Here's how the part is built. I have some questions about the finished solid (model axes, mm). A direction names the side the tool comes from. Give positions to 0.01 mm unless a question says otherwise; leave off trailing zeros. Loops run counter-clockwise (first coordinate to the right, second up) from the corner with the lowest first, then second, coordinate; pieces in that order, holes last.
Q1. Suppose I cut it at C-C (x = -15.5). List the corners of the cut face in (y, z) for me, and give its area (3 significant figures).
Q2. I need wall thicknesses on probe 1 along Y at (x, z) = (-25, 2.2); probe 2 along Y at (x, z) = (-15.5, 0.3); probe 3 along X at (y, z) = (34, 2.4) (3 decimals). Which ranges of each line are inside material? Lowest first, please.
Q3. Thinking about a two-plate mould opening in Y: for faces 1 (the face through (-16.51, -2.19, 1.25)), 2 (the face through (-2, 40.005, 1)), 3 (the face through (-22, -0.889, 1)), 4 (the face through (2.54, 19, 1)), which applies, pulls with the +Y half, pulls with the -Y half, needs draft (parallel to the pull), parting line crosses it, or undercut?
Q4. For faces 5 (the face through (0, -2, 1)), 6 (the face through (1, -3.175, 1)), 7 (the face through (-20, 3.81, 1)), which set-ups out of +Z, -Z, +X, -X, +Y, -Y let a thin tool reach every point of the face, with its end or its side?
Q5. I'm going to push flat-ended pins straight in: P1, Ø1.3, axis at x = -21.5, z = 1, coming from the +Y side; P2, Ø0.8, axis at y = 28, z = 1.5, coming from the -X side (3 decimals); P3, Ø0.8, axis at x = -10, z = 1, coming from the -Y side. Where does each tip first touch, or does it pass through?
Q6. Suppose I cut it at B-B (y = 36.5). List the corners of the cut face in (x, z) for me (3 decimals), and give its area (3 significant figures).
```python
from build123d import *

# Parameters (mm, degrees)
F1_DEPTH = 2.54


with BuildPart() as f1:
    # F0 (on Top) → F1 (new body)
    with BuildSketch(Plane.XY):
        with BuildLine():
            Line((2.54, 40.005), (-6.985, 40.005))
            Line((-6.985, 40.005), (-6.985, 10.16))
            ThreePointArc((-6.985, 10.16), (-8.844872, 5.669872), (-13.335, 3.81))
            Line((-13.335, 3.81), (-26.67, 3.81))
            ThreePointArc((-26.67, 3.81), (-30.2895, 0.1905), (-26.67, -3.429))
            Line((-26.67, -3.429), (-17.78, -3.429))
            ThreePointArc((-17.78, -3.429), (-16.51, -2.159), (-17.78, -0.889))
            Line((-17.78, -0.889), (-25.4, -0.889))
            Line((-25.4, -0.889), (-25.4, 0))
            Line((-25.4, 0), (0, 0))
            Line((0, 0), (0, -3.175))
            Line((0, -3.175), (1.2192, -3.175))
            ThreePointArc((1.2192, -3.175), (2.153147, -2.788147), (2.54, -1.8542))
            Line((2.54, -1.8542), (2.54, 40.005))
        make_face()
    extrude(amount=F1_DEPTH)


solid = f1.part
```
Solutions:
1. outline: (0, 0) - (3.81, 0) - (3.81, 2.54) - (0, 2.54) - close
1. area: 9.68 mm2
2. probe 1: y = -3.43 to -0.89, 0 to 3.81
2. probe 2: y = 0 to 3.81
2. probe 3: x = -6.985 to 2.54
3. face 1: undercut
3. face 2: pulls with the +Y half
3. face 3: undercut
3. face 4: needs draft
4. face 5: +Z, -Z, -Y
4. face 6: +Z, -Z, +X, -Y
4. face 7: +Z, -Z, -X, +Y
5. P1: stops at y = 3.81
5. P2: stops at x = -6.985
5. P3: stops at y = 0
6. outline: (-6.985, 0) - (2.54, 0) - (2.54, 2.54) - (-6.985, 2.54) - close
6. area: 24.2 mm2
